Check sheet for the modelled part. Datum: model origin and axes. Units: mm. A direction names the side the tool comes from. Round coordinates to 2 decimals unless told otherwise and drop trailing zeros. Order: outer loops, then holes, each group sorted by start corner. A loop starts at its lowest first (then second) coordinate and runs counter-clockwise, first axis right, second up.
Autodesk Inventor part; units mm, degrees
ref_plane "FDT_CYLINDER_XY" through (0, 0, -4) normal (0, 0, 1) x (1, 0, 0)
ref_plane "FDT_CYLINDER_YZ" through (0, 0, -4) normal (1, 0, 0) x (0, 1, 0)
ref_plane "FDT_CYLINDER_ZX" through (0, 0, -4) normal (0, 1, 0) x (0, 0, 1)
sketch "Sketch_1" plane through (0, 0, 0) normal (1, 0, 0) x (0, 1, 0)
  line L0 (0, -4) -> (0, 4)
  line L1 (0, 4) -> (18, 4)
  line L2 (18, 4) -> (18, 3.5)
  line L3 (18, 3.5) -> (21, 3.5)
  line L4 (21, 3.5) -> (21, -4)
  line L5 (21, -4) -> (0, -4)
  line L6 (0, -4) -> (0, 4)
revolve "Revolution1" add sketch "Sketch_1" angle 360 about axis through (0, 0, -4) along (0, 0, -1)
sketch "Sketch_2" plane through (0, 0, 0) normal (1, 0, 0) x (0, 1, 0)
  line L0 (0, -4) -> (0, 4)
  line L1 (0, 4) -> (15, 4)
  line L2 (15, 4) -> (14.188, 3.5312)
  line L3 (14.188, 3.5312) -> (14.188, -3.188)
  line L4 (14.188, -3.188) -> (15, -4)
  line L5 (15, -4) -> (0, -4)
  line L6 (0, -4) -> (0, 4)
revolve "Revolution2" cut sketch "Sketch_2" angle 360 about axis through (0, 0, -4) along (0, 0, -1)
thread "Thread1"
sketch "Sketch_6" plane through (0, 0, 0) normal (1, 0, 0) x (0, 1, 0)
  line L0 (0, -6) -> (0, -4)
  line L1 (0, -4) -> (18, -4)
  line L2 (18, -4) -> (18, -3.5)
  line L3 (18, -3.5) -> (21, -3.5)
  line L4 (21, -3.5) -> (21, -6)
  line L5 (21, -6) -> (0, -6)
  line L6 (0, -6) -> (0, -4)
revolve "Revolution3" cut sketch "Sketch_6" angle 360 about axis through (0, 0, -6) along (0, 0, -1)
sketch "Sketch_3" plane through (0, 0, 0) normal (0, 0, 1) x (1, 0, 0)
  circle A0 centre (0, 0) radius 25.2
  line L0 (-20.7846, 3) -> (-18.5, 3)
  line L1 (-18.5, 3) -> (-18.5, -3)
  line L2 (-18.5, -3) -> (-20.7846, -3)
  arc A1 (-20.7846, -3) -> (-3, -20.7846) centre (0, 0) ccw
  line L3 (-3, -20.7846) -> (-3, -18.5)
  line L4 (-3, -18.5) -> (3, -18.5)
  line L5 (3, -18.5) -> (3, -20.7846)
  arc A2 (3, -20.7846) -> (20.7846, -3) centre (0, 0) ccw
  line L6 (20.7846, -3) -> (18.5, -3)
  line L7 (18.5, -3) -> (18.5, 3)
  line L8 (18.5, 3) -> (20.7846, 3)
  arc A3 (20.7846, 3) -> (3, 20.7846) centre (0, 0) ccw
  line L9 (3, 20.7846) -> (3, 18.5)
  line L10 (3, 18.5) -> (-3, 18.5)
  line L11 (-3, 18.5) -> (-3, 20.7846)
  arc A4 (-3, 20.7846) -> (-20.7846, 3) centre (0, 0) ccw
extrude "Extrusion1" cut sketch "Sketch_3" along normal mid plane 8
ref_plane "FDT_CYLINDER_XY" through (0, 0, -4) normal (0, 0, 1) x (1, 0, 0)
ref_plane "FDT_CYLINDER_YZ" through (0, 0, -4) normal (1, 0, 0) x (0, 1, 0)
ref_plane "FDT_CYLINDER_ZX" through (0, 0, -4) normal (0, 1, 0) x (0, 0, 1)
ref_plane "NUT_XY" through (0, 0, 4) normal (0, 0, -1) x (1, 0, 0)
ref_plane "NUT_YZ" through (0, 0, 4) normal (1, 0, 0) x (0, -1, 0)
ref_plane "NUT_ZX" through (0, 0, 4) normal (0, -1, 0) x (0, 0, -1)
properties part number "3753 M30x1.5"
Item 1: Access from +Z, -Z, +X, -X, +Y, -Y to the whole of each face (thin tool, end or side, straight path). Record for faces 1 (the flat face through (14, 12, 3.5)), 2 (the flat face through (-3, 20, 0)), 3 (the flat face through (-3, -20, 0)).
Answer:
face 1: +Z
face 2: +Z, -Z, +Y
face 3: +Z, -Z, -Y
Item 2: Sectioned sample at D-D (x = -16). Record the cut outline in (y, z), and give its area (3 significant figures).
Answer:
outline: (-13.6, -3.5) - (-8.25, -3.5) - (-8.25, -4) - (8.25, -4) - (8.25, -3.5) - (13.6, -3.5) - (13.6, 3.5) - (8.25, 3.5) - (8.25, 4) - (-8.25, 4) - (-8.25, 3.5) - (-13.6, 3.5) - close
area: 207 mm2
Item 3: Sectioned sample at C-C (z = -2). Record the cut outline in (x, y).
Answer:
outline: (-20.78, -3) arc R21 ccw to (-3, -20.78) - (-3, -18.5) - (3, -18.5) - (3, -20.78) arc R21 ccw to (20.78, -3) - (18.5, -3) - (18.5, 3) - (20.78, 3) arc R21 ccw to (3, 20.78) - (3, 18.5) - (-3, 18.5) - (-3, 20.78) arc R21 ccw to (-20.78, 3) - (-18.5, 3) - (-18.5, -3) - close; hole circle Ø28.38 at (0, 0)
Item 4: Scan lines: line 1 along X through (y, z) = (0, -1); line 2 along Z through (x, y) = (-14, 11.5); line 3 along Y through (x, z) = (-0.5, 2.25). Record each from-to range of solid material in increasing order.
Answer:
line 1: x = -18.5 to -14.19, 14.19 to 18.5
line 2: z = -3.5 to 3.5
line 3: y = -18.5 to -14.18, 14.18 to 18.5
Item 5: Go/stop test with flat-tipped pins: P1, Ø1, axis at x = 6, z = -2.5, coming from the -Y side; P2, Ø4, axis at x = -10, z = 3, coming from the -Y side; P3, Ø1, axis at x = -9, z = 1.5, coming from the +Y side; P4, Ø5, axis at x = 11.5, y = 7, coming from the +Z side. Record where each tip stops, or that it passes through.
Answer:
P1: stops at y = -20.27
P2: stops at y = -19.42
P3: stops at y = 19.2
P4: stops at z = 4
Item 6: Release check for a two-part mould opening along X. For faces 4 (the flat face through (14, 12, -3.5)), 5 (the cylindrical face through (14.72, 14.98, -0.05)), 6 (the flat face through (0, -18.5, 0)) record: released by +X, released by -X, zero draft, split by the parting line, or undercut.
Answer:
face 4: zero draft
face 5: released by +X
face 6: undercut
Item 7: Sectioned sample at A-A (y = 0). Record the cut outline in (x, z).
Answer:
outline: (-18.5, -3.5) - (-18, -3.5) - (-18, -4) - (-15, -4) - (-14.19, -3.19) - (-14.19, 3.53) - (-15, 4) - (-18, 4) - (-18, 3.5) - (-18.5, 3.5) - close; (14.19, -3.19) - (15, -4) - (18, -4) - (18, -3.5) - (18.5, -3.5) - (18.5, 3.5) - (18, 3.5) - (18, 4) - (15, 4) - (14.19, 3.53) - close
